Could you check a few things on this drawing? It's one solid part, dimensions in mm from its lowest x, y, z. A direction names the side the tool comes from. Give positions to 0.01 mm unless a question says otherwise; leave off trailing zeros. Order: outer loops, then holes, each group sorted by start corner. A loop starts at its lowest first (then second) coordinate and runs counter-clockwise, first axis right, second up. Notation, with made-up numbers: M -0.75,14 L 51.25,14 A13 ccw 51.25,22 Z; hole C -33.5,-28.5 d8. An arc over 180 degrees is marked long. Use one line per item in the form item = value. Start each with the question number.
1. I want a section at D-D, the plane z = 14. List the corners of the cut face in (x, y) for me, and give its area (3 significant figures).
2. We'd pull the mould along Z, two halves only. Please class the marked faces 1, 2 and 3: +Z half, -Z half, draft (parallel to the pull), parting line (faces both ways), or undercut.
3. Will these pins go through, and if not, where does the flat tip stop? P1, Ø4.5, axis at x = 10, z = 9, coming from the +Y side; P2, Ø5.5, axis at x = 9.5, z = 6.5, coming from the +Y side.
4. I need wall thicknesses on L1, parallel to Z at x = 1.8, y = 10; L2, parallel to X at y = 6, z = 12.75; L3, parallel to Y at x = 1.7, z = 9. Which ranges of each line are inside material? Lowest first, please.
5. I want a section at A-A, the plane x = 10. List the corners of the cut face in (y, z) for me, and give its area (3 significant figures).
6. For the marked faces 4 and 5, which set-ups out of +Z, -Z, +X, -X, +Y, -Y let a thin tool reach every point of the face, with its end or its side?
7. I want a section at B-B, the plane z = 9. List the corners of the cut face in (x, y) for me.
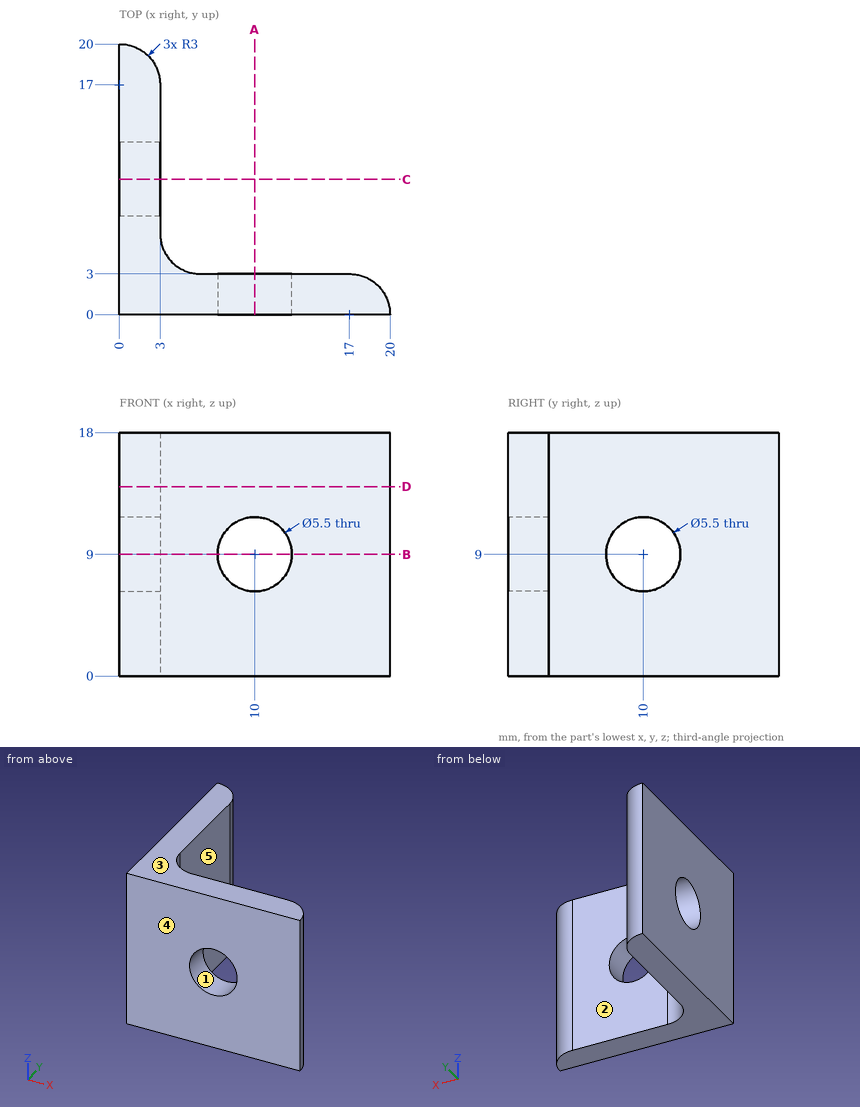
Check result:
q1.outline = M 0,0 L 20,0 A3 ccw 17,3 L 6,3 A3 cw 3,6 L 3,17 A3 ccw 0,20 Z
q1.area = 109 mm2
q2.face_1 = undercut
q2.face_2 = draft
q2.face_3 = +Z half
q3.P1 = through
q3.P2 = 3
q4.L1 = 0 to 6.25, 11.75 to 18
q4.L2 = 0 to 3
q4.L3 = 0 to 7.25, 12.75 to 19.47
q5.outline = M 0,0 L 3,0 L 3,6.25 L 0,6.25 Z; M 0,11.75 L 3,11.75 L 3,18 L 0,18 Z
q5.area = 37.5 mm2
q6.face_4 = +Z, -Z, +X, -X, -Y
q6.face_5 = +Z, -Z, +X, +Y
q7.outline = M 0,0 L 7.25,0 L 7.25,3 L 6,3 A3 cw 3,6 L 3,7.25 L 0,7.25 Z; M 0,12.75 L 3,12.75 L 3,17 A3 ccw 0,20 Z; M 12.75,0 L 20,0 A3 ccw 17,3 L 12.75,3 Z
